Geometry: final body of the model. Coordinates: model frame, mm. A direction names the side the tool comes from. Round coordinates to 2 decimals unless told otherwise and drop trailing zeros. Write each loop counter-clockwise with the first axis right and the second up, starting at its lowest first coordinate (ties: lowest second). Pieces come first, ordered by that corner, then holes. Notation, with made-up numbers: (23.5, 86.25) -> (36.5, 86.25) arc R12 cw to (36.5, 99.25) -> close; hole circle Ø3 at (25, -16). An arc over 180 degrees is marked (long way). One line per item, written item: value. Start each with the question number.
from build123d import *

# Parameters (mm, degrees)
F1_DEPTH    = 25.4
F2_T1_DEPTH = 76.2
F3_R        = 12.69999
F6_DEPTH    = 25.4
F4_R        = 6.35
F7_DEPTH    = 25.4


# Not quite as in the source:
# - a fillet or chamfer that OpenCascade refuses, or shapes differently, is made with other operations: its cross-section is extruded or revolved along the edge and cut away or added
# - a fillet or chamfer is up to 0.001 mm smaller than in the source, because OpenCascade refuses the exact size


with BuildPart() as f1:
    # F0 (on Right) → F1 (new body)
    with BuildSketch(Plane.YZ):
        Polygon((-57.15, 0), (0, 0), (0, 44.45), (-12.7, 44.45), (-12.7, 12.7), (-57.15, 12.7), align=None)
    extrude(amount=F1_DEPTH)

    # F2: fillet of radius 12.7 on 2 edges, made by hand

    # F2_s2 → F2_t1 (cut)
    with BuildSketch(Plane.XZ.offset(-31.75)):
        with BuildLine():
            ThreePointArc((12.7, 44.45), (3.7197438789, 40.7302561211), (0, 31.75))
            Line((0, 31.75), (0, 44.45))
            Line((0, 44.45), (12.7, 44.45))
        make_face()
        with BuildLine():
            ThreePointArc((12.7, 44.45), (21.6802561211, 40.7302561211), (25.4, 31.75))
            Line((25.4, 31.75), (25.4, 44.45))
            Line((25.4, 44.45), (12.7, 44.45))
        make_face()
    extrude(amount=F2_T1_DEPTH, mode=Mode.SUBTRACT)

    # F3 (radius 12.7 in the source; OpenCascade refuses exactly that, so slightly less here)
    f3_edges = [f1.edges().sort_by_distance(p)[0] for p in [
        (25.4, -57.15, 6.35),
        (0, -57.15, 6.35),
    ]]
    fillet(f3_edges, radius=F3_R)

    # F5 (on face) → F6 (cut)
    with BuildSketch(Plane(origin=(0, 0, 0), x_dir=(-1, 0, 0), z_dir=(0, 1, 0))):
        with BuildLine():
            ThreePointArc((-19.05, 31.75), (-12.7, 25.4), (-6.35, 31.75))
            ThreePointArc((-6.35, 31.75), (-12.7, 38.1), (-19.05, 31.75))
        make_face()
        with BuildLine():
            ThreePointArc((-19.05, 31.75), (-12.7, 38.1), (-6.35, 31.75))
            Line((-6.35, 31.75), (-6.35, 42.7485226281))
            ThreePointArc((-6.35, 42.7485226281), (-9.4129981272, 44.0172579939), (-12.7, 44.45))
            ThreePointArc((-12.7, 44.45), (-15.9870018728, 44.0172579939), (-19.05, 42.7485226281))
            Line((-19.05, 42.7485226281), (-19.05, 31.75))
        make_face()
    extrude(amount=-F6_DEPTH, mode=Mode.SUBTRACT)

    # F4 (on face) → F7 (cut)
    with BuildSketch(Plane.XY.offset(12.7)):
        with Locations((12.7, -44.45)):
            Circle(F4_R)
        with Locations((12.7, -25.4)):
            Circle(F4_R)
    extrude(amount=-F7_DEPTH, mode=Mode.SUBTRACT)


solid = f1.part
(1) Section query C-C (y = -8). Output: boundary loops of the cut face in (x, z), and give its area (3 significant figures).
(2) Set-up query: faces 4 (the face through (7.66, -29.26, 6.44)), 5 (the face through (19.05, -6, 37)), 6 (the face through (13, -12.7, 25)). Return all of +Z, -Z, +X, -X, +Y, -Y with unobstructed straight access to the full face (end or side cutting, diameter ignored); none if empty.
(3) Pull-direction query (X, two-part tool) for faces 1 (the face through (11.873, -38.154, 6.439)), 2 (the face through (25.4, -18, 9)), 3 (the face through (1.75, -6.26, 38.18)); classes: pulls with the +X half, pulls with the -X half, needs draft (parallel to the pull), parting line crosses it, or undercut.
(4) Line query: probe 1 along Y at (x, z) = (12.7, 4.5); probe 2 along Z at (x, y) = (16.75, -14.5); probe 3 along Y at (x, z) = (13.5, 12.5). Output: solid intervals per line, ascending.
(5) Pin query (flat end, axial travel): pin 1 (1 mm diameter, centred on y = -11, z = 33.5, fed in from +X); pin 2 (3.5 mm diameter, centred on y = -9, z = 37, fed in from -X); pin 3 (5 mm diameter, centred on y = -50, z = 16, fed in from -X); pin 4 (7.5 mm diameter, centred on x = 8, z = 28.5, fed in from -Y). Return the tip coordinate at first contact, or that it passes through.
(6) Section query D-D (z = 31). Output: boundary loops of the cut face in (x, y), and give its area (3 significant figures).
(7) Section query B-B (x = 16). Output: boundary loops of the cut face in (y, z), and give its area (3 significant figures).
(8) Section query A-A (y = -25.4). Output: boundary loops of the cut face in (x, z), and give its area (3 significant figures).
Results list:
1. outline: (0, 0) -> (25.4, 0) -> (25.4, 31.75) arc R12.7 ccw to (19.05, 42.75) -> (19.05, 31.75) arc R6.35 cw to (6.35, 31.75) -> (6.35, 42.75) arc R12.7 ccw to (0, 31.75) -> close
1. area: 842 mm^2
2. face 4: +Z, -Z
2. face 5: +Z, +Y, -Y
2. face 6: +Z, +X, -X, -Y
3. face 1: undercut
3. face 2: pulls with the +X half
3. face 3: pulls with the -X half
4. probe 1: y = -57.15 to -50.8, -38.1 to -31.75, -19.05 to 0
4. probe 2: z = 0 to 12.7
4. probe 3: y = -57.12 to -50.75, -38.15 to -31.7, -19.1 to 0
5. pin 1: stops at x = 25.34
5. pin 2: stops at x = 0.49
5. pin 3: passes through
5. pin 4: stops at y = -12.7
6. outline: (0, -12.7) -> (6.39, -12.7) -> (6.39, 0) -> (0, 0) -> close; (19.01, -12.7) -> (25.4, -12.7) -> (25.4, 0) -> (19.01, 0) -> close
6. area: 162 mm^2
7. outline: (-56.71, 0) -> (-49.88, 0) -> (-49.88, 12.7) -> (-56.71, 12.7) -> close; (-39.02, 0) -> (-30.83, 0) -> (-30.83, 12.7) -> (-39.02, 12.7) -> close; (-19.97, 0) -> (0, 0) -> (0, 26.32) -> (-12.7, 26.32) -> (-12.7, 12.7) -> (-19.97, 12.7) -> close
7. area: 618 mm^2
8. outline: (0, 0) -> (6.35, 0) -> (6.35, 12.7) -> (0, 12.7) -> close; (19.05, 0) -> (25.4, 0) -> (25.4, 12.7) -> (19.05, 12.7) -> close
8. area: 161 mm^2
